CAD build for the part. Positions are in the model's coordinates, mm. A direction names the side the tool comes from. Round coordinates to 2 decimals unless told otherwise and drop trailing zeros. Loops run counter-clockwise (first coordinate to the right, second up) from the corner with the lowest first, then second, coordinate; pieces in that order, holes last.
```python
from build123d import *

# Parameters (mm, degrees)
F1_DEPTH = 3.175


with BuildPart() as f1:
    # F0 (on Right) → F1 (new body, symmetric)
    with BuildSketch(Plane.YZ):
        Polygon((50.8, -58.581289), (0, -58.581289), (-25.4, -58.581289), (-25.4, -64.931289), (50.8, -64.931289), align=None)
        Polygon((-25.4, -58.581289), (0, -58.581289), (50.8, -58.581289), (76.2, -58.581289), (101.6, -34.879341), (101.6, 90.705617), (76.2, 98.488349), (17.829527, 98.488349), (-50.8, -58.581289), align=None)
    extrude(amount=F1_DEPTH, both=True)


solid = f1.part
```
Item 1: Cut at C-C, the plane y = 68.5. Give the cut face in (x, z) (3 decimals), plus the area to 3 significant figures.
Answers follow:
outline: (-3.175, -58.581) - (3.175, -58.581) - (3.175, 98.488) - (-3.175, 98.488) - close
area: 997 mm2
Item 2: Probe line 1 (Z direction, x = -0.25, y = 72.5); line 2 (Z direction, x = -0.25, y = -30); line 3 (Y direction, x = 2.5, z = 50.5). List the from-to ranges inside material, lowest first.
Answers follow:
line 1: z = -58.58 to 98.49
line 2: z = -58.58 to -10.98
line 3: y = -3.14 to 101.6
Item 3: Flat gauge pins, fed straight in: P1, Ø1.5, axis at x = 1.5, z = -38, coming from the -Y side (3 decimals); P2, Ø1.9, axis at x = -1, y = 68, coming from the -Z side; P3, Ø1.9, axis at x = -1, z = -62, coming from the +Y side. Where does each tip first touch, or does it go through?
Answers follow:
P1: stops at y = -42.135
P2: stops at z = -58.58
P3: stops at y = 50.8
Item 4: Cut at B-B, the plane z = -20.5. Give the cut face in (x, y) (3 decimals), plus the area to 3 significant figures.
Answers follow:
outline: (-3.175, -34.161) - (3.175, -34.161) - (3.175, 101.6) - (-3.175, 101.6) - close
area: 862 mm2
Item 5: Cut at A-A, the plane x = 1.25. Give the cut face in (y, z).
Answers follow:
outline: (-50.8, -58.58) - (-25.4, -58.58) - (-25.4, -64.93) - (50.8, -64.93) - (50.8, -58.58) - (76.2, -58.58) - (101.6, -34.88) - (101.6, 90.71) - (76.2, 98.49) - (17.83, 98.49) - close
Item 6: 3-axis set-ups, long thin cutter, end or side, ignore diameter. For faces 1 (the flat face through (0, 101.6, 27)), 2 (the flat face through (0, -38, -58.581)), 3 (the flat face through (0, 50.8, -62)): which of +Z, -Z, +X, -X, +Y, -Y reach the whole face in a straight line?
Answers follow:
face 1: +Z, -Z, +X, -X, +Y
face 2: -Z, +X, -X, -Y
face 3: -Z, +X, -X, +Y
